Autodesk Inventor part; units mm, degrees
ref_plane "Work Plane1" through (3, 20, 0) normal (0.7071, 0.7071, 0) x (0, 0, 1)
ref_plane "YZ Plane" through (0, 0, 0) normal (1, 0, 0) x (0, 1, 0)
ref_plane "XZ Plane" through (0, 0, 0) normal (0, 1, 0) x (-1, 0, 0)
sketch "Sketch2" plane through (0, 0, 0) normal (0, 0, 1) x (1, 0, 0)
  line L0 (3, 20) -> (0, 20)
  line L1 (0, 20) -> (0, 0)
  line L2 (0, 0) -> (20, 0)
  line L3 (20, 0) -> (20, 3)
  line L4 (20, 3) -> (3, 3)
  line L5 (3, 3) -> (3, 20)
  dimension "d0" = 20
  dimension "d1" = 3
extrude "Extrusion1" add sketch "Sketch2" along normal blind 17
ref_plane "Work Plane1" through (3, 20, 0) normal (0.7071, 0.7071, 0) x (0, 0, 1)
sketch "Sketch3" plane through (3, 20, 0) normal (0.7071, 0.7071, 0) x (0, 0, 1)
  line L0 (0, 24.0416) -> (17, 24.0416)
  line L1 (17, 0) -> (15, 0)
  line L2 (15, 0) -> (15, 24.0416)
  line L3 (15, 24.0416) -> (17, 24.0416)
  line L4 (17, 24.0416) -> (17, 0)
  line L5 (0, 24.0416) -> (2, 24.0416)
  line L6 (2, 24.0416) -> (2, 0)
  line L7 (2, 0) -> (0, 0)
  line L8 (0, 0) -> (0, 24.0416)
  point P0 (0, 12.0208)
  dimension "d4" = 2
  dimension "d5" = 2
extrude "Extrusion2" add sketch "Sketch3" against normal up to next
sketch "Sketch4" plane through (3, 3, 2) normal (0, 1, 0) x (1, 0, 0)
  arc A0 (5, -3.5) -> (5, -9.5) centre (5, -6.5) ccw
  arc A1 (8, -9.5) -> (8, -3.5) centre (8, -6.5) ccw
  line L0 (8, -3.5) -> (5, -3.5)
  line L1 (8, -9.5) -> (5, -9.5)
  line L2 (-3, 2) -> (-3, -15)
  point P0 (-3, -6.5)
  point P1 (-3, -6.5)
  dimension "d8" = 6
  dimension "d9" = 6
  dimension "d10" = 3
  dimension "d11" = 8
extrude "Extrusion3" cut sketch "Sketch4" against normal blind 6
pattern_circular "Circular Pattern2" count 2 over 90 about axis through (0, 0, 0) along (0, 0, 1) of "Extrusion3"
equation "\"d5\" = d4"
equation "\"d9\" = d8"
properties part number "20x20 90 Gusset"
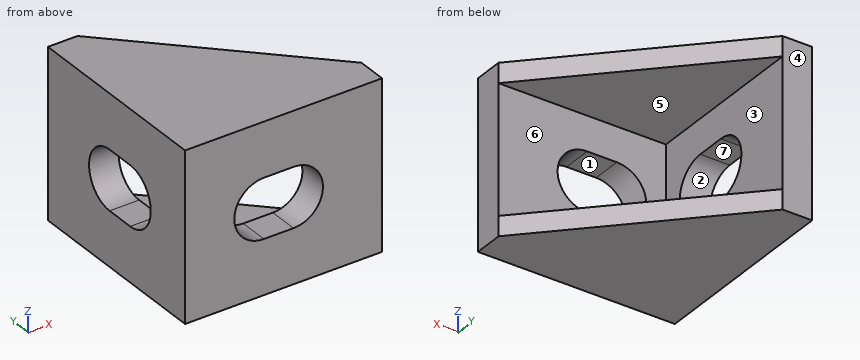
Verification items for the finished model (mm, model axes). Face numbers are marked on the shaded views. A direction names the side the tool comes from. Round coordinates to 2 decimals unless told otherwise and drop trailing zeros. Loops run counter-clockwise (first coordinate to the right, second up) from the corner with the lowest first, then second, coordinate; pieces in that order, holes last. Notation, with made-up numbers: (20.25, 50) - (63.25, 50) arc R30 ccw to (63.25, 81) - close; hole circle Ø4 at (65.25, 20.5). An arc over 180 degrees is marked (long way). Use a Markdown table: item, result. Add a question column.
1. Section check B-B, the plane x = 2.25. Record the boundary of the cut face in (y, z), plus the area to 3 significant figures.
2. Section check D-D, the plane y = 4.5. Record the boundary of the cut face in (x, z).
3. Release check for a two-part mould opening along Y. For the marked faces 5, 6 and 7 record: released by +Y, released by -Y, zero draft, split by the parting line, or undercut.
4. Gauge pin test, flat ends, axial feed: pin 1 (5 mm diameter, centred on y = 10, z = 3, fed in from +X); pin 2 (3 mm diameter, centred on y = 6.5, z = 13, fed in from +X); pin 3 (5 mm diameter, centred on x = 13, z = 8, fed in from +Y). Record the tip position at first contact, or that the pin passes through.
5. Section check A-A, the plane y = 9.75. Record the boundary of the cut face in (x, z).
6. Access from +Z, -Z, +X, -X, +Y, -Y to the whole of each face (thin tool, end or side, straight path). Record for the marked faces 1, 2, 3 and 4.
7. Thickness scan on probe 1 along Z at (x, y) = (14.25, 7.25); probe 2 along X at (y, z) = (19.25, 8.75). Record the ranges inside material, lowest first. Write a range as [from, to].
Checks:
| question | item | result |
|---|---|---|
| 1 | outline | (0, 0) - (20, 0) - (20, 17) - (0, 17) - close; hole (8, 5.5) - (11, 5.5) arc R3 ccw to (11, 11.5) - (8, 11.5) arc R3 ccw to start |
| 1 | area | 294 mm^2 |
| 2 | outline | (0, 0) - (18.5, 0) - (18.5, 2) - (3, 2) - (3, 15) - (18.5, 15) - (18.5, 17) - (0, 17) - close |
| 3 | face 5 | zero draft |
| 3 | face 6 | released by +Y |
| 3 | face 7 | undercut |
| 4 | pin 1 | stops at x = 15.29 |
| 4 | pin 2 | stops at x = 3 |
| 4 | pin 3 | stops at y = 3 |
| 5 | outline | (0, 0) - (13.25, 0) - (13.25, 2) - (3, 2) - (3, 5.5) - (0, 5.5) - close; (0, 11.5) - (3, 11.5) - (3, 15) - (13.25, 15) - (13.25, 17) - (0, 17) - close |
| 6 | face 1 | +Y, -Y |
| 6 | face 2 | +X, -X |
| 6 | face 3 | +X, +Y |
| 6 | face 4 | +Z, -Z, +X, -X, +Y |
| 7 | probe 1 | z = [0, 2], [15, 17] |
| 7 | probe 2 | x = [0, 3] |
